Can you work these out from the model? Positions are in its coordinate system, mm. Give positions to 0.01 mm unless a question says otherwise; leave off trailing zeros. Loops run counter-clockwise (first coordinate to the right, second up) from the corner with the lowest first, then second, coordinate; pieces in that order, holes last. Notation, with made-up numbers: (2, 80.25) -> (28, 80.25) arc R24 ccw to (28, 91.25) -> close; hole circle Ø3 at (85.5, -10.5). An arc over 180 degrees is marked (long way). Return JSON: item names as keys, results as strings. Group by question number.
Q1. Will these pins go through, and if not, where does the flat tip stop? pin 1 (1 mm diameter, centred on y = -1, z = 1.5, fed in from -X); pin 2 (0.6 mm diameter, centred on y = -1, z = 1, fed in from +X).
Q2. Suppose I cut it at B-B, the plane z = 1.2. Please give me the cut outline in (x, y).
Q3. I need wall thicknesses on line 1 along Y through (x, z) = (13, 0.3); line 2 along X through (y, z) = (2, 1.3); line 3 along X through (y, z) = (1.5, 1.25). Which ranges of each line are inside material? Lowest first, please. Write a range as [from, to].
Q4. Suppose I cut it at D-D, the plane y = 6. Please give me the cut outline in (x, z), and give its area (3 significant figures).
Q5. Thinking about a two-plate mould opening in X: for faces 1 (the flat face through (69, -8, 1)), 2 (the flat face through (-1, -5, 2)), 3 (the cylindrical face through (-79.53, -7.38, 0.99)), which applies, pulls with the +X half, pulls with the -X half, needs draft (parallel to the pull), parting line crosses it, or undercut?
Q6. Suppose I cut it at C-C, the plane x = -47. Please give me the cut outline in (y, z).
Q7. Suppose I cut it at A-A, the plane x = 73.5. Please give me the cut outline in (y, z).
```python
from build123d import *

# Parameters (mm, degrees)
F0_W        = 193
F0_H        = 20
F1_DEPTH    = 2
F2_W        = 5
F2_H        = 5
F2_W_2      = 167
F3_DEPTH    = 25
F4_SIZE2    = 14.99999
F4_SIZE     = 9.99999
F5_W        = 6
F5_H        = 4
F6_DEPTH    = 25
F7_T1_DEPTH = 106.0916256943
F8_DEPTH    = 10.6


# Not quite as in the source:
# - a fillet or chamfer that OpenCascade refuses, or shapes differently, is made with other operations: its cross-section is extruded or revolved along the edge and cut away or added
# - a fillet or chamfer is up to 0.001 mm smaller than in the source, because OpenCascade refuses the exact size


with BuildPart() as f1:
    # F0 (on Top) → F1 (new body)
    with BuildSketch(Plane.XY):
        Rectangle(F0_W, F0_H)
    extrude(amount=F1_DEPTH)

    # F2 (on face) → F3 (cut)
    with BuildSketch(Plane.XY.offset(2)):
        with Locations((94, 0)):
            Rectangle(F2_W, F2_H)
        with Locations((-3, 0)):
            Rectangle(F2_W_2, F2_H)
    extrude(amount=-F3_DEPTH, mode=Mode.SUBTRACT)

    # F4 (size 10 and 15 in the source; OpenCascade refuses exactly that, so slightly less here)
    f4_edges = [f1.edges().sort_by_distance(p)[0] for p in [
        (-96.5, 10, 1),
        (-96.5, -10, 1),
    ]]
    f4_side = f1.faces().sort_by_distance((-96.5, 0, 1))[0]
    chamfer(f4_edges, length=F4_SIZE, length2=F4_SIZE2, reference=f4_side)

    # F5 (on face) → F6 (cut)
    with BuildSketch(Plane.XY.offset(2)):
        with Locations((93.5, -8)):
            Rectangle(F5_W, F5_H)
        Polygon((61.5, -10), (76.5, -10), (76.5, -6), align=None)
    extrude(amount=-F6_DEPTH, mode=Mode.SUBTRACT)

    # F7: fillet of radius 69.147644117 on 2 edges, made by hand

    # F7_s2 → F7_t1 (cut)
    with BuildSketch(Plane.XY.offset(-52.0458128472)):
        with BuildLine():
            ThreePointArc((-96.5, -1e-05), (-79.2757127961, -7.4530977113), (-60.6816848611, -10))
            Line((-60.6816848611, -10), (-81.50001, -10))
            Line((-81.50001, -10), (-96.5, -1e-05))
        make_face()
        with BuildLine():
            ThreePointArc((-96.5, 1e-05), (-79.2757127961, 7.4530977113), (-60.6816848611, 10))
            Line((-60.6816848611, 10), (-81.50001, 10))
            Line((-81.50001, 10), (-96.5, 1e-05))
        make_face()
    extrude(amount=F7_T1_DEPTH, mode=Mode.SUBTRACT)

    # F8 (add): a face of the model
    f8_faces = [f1.faces().sort_by_distance(p)[0] for p in [
        (-86.5, 0, 1),
    ]]
    extrude(f8_faces, amount=F8_DEPTH)


solid = f1.part
```
Ans:
{
 "1": {"pin 1": "stops at x = -95.66", "pin 2": "stops at x = 91.5"},
 "2": {"outline": "(-96.5, 0) arc R69.15 ccw to (-60.68, -10) -> (61.5, -10) -> (76.5, -6) -> (76.5, -10) -> (90.5, -10) -> (90.5, -6) -> (96.5, -6) -> (96.5, -2.5) -> (91.5, -2.5) -> (91.5, 2.5) -> (96.5, 2.5) -> (96.5, 10) -> (-60.68, 10) arc R69.15 ccw to start; hole (-75.9, -2.5) -> (80.5, -2.5) -> (80.5, 2.5) -> (-75.9, 2.5) -> close"},
 "3": {"line 1": "y = [-10, -2.5], [2.5, 10]", "line 2": "x = [-92.97, -75.9], [80.5, 91.5]", "line 3": "x = [-93.9, -75.9], [80.5, 91.5]"},
 "4": {"outline": "(-83.86, 0) -> (96.5, 0) -> (96.5, 2) -> (-83.86, 2) -> close", "area": "361 mm^2"},
 "5": {"face 1": "undercut", "face 2": "needs draft", "face 3": "pulls with the -X half"},
 "6": {"outline": "(-10, 0) -> (-2.5, 0) -> (-2.5, 2) -> (-10, 2) -> close; (2.5, 0) -> (10, 0) -> (10, 2) -> (2.5, 2) -> close"},
 "7": {"outline": "(-6.8, 0) -> (-2.5, 0) -> (-2.5, 2) -> (-6.8, 2) -> close; (2.5, 0) -> (10, 0) -> (10, 2) -> (2.5, 2) -> close"}
}
